Geometry: see drawing. Coordinates: mm, zero at the bounding-box minimum. Give positions to 0.01 mm unless a question says otherwise; leave off trailing zeros. Order: outer loops, then holes, each group sorted by start corner. A loop starts at its lowest first (then second) coordinate and runs counter-clockwise, first axis right, second up. Notation, with made-up numbers: (36, 62.25) -> (49, 62.25) arc R32 cw to (49, 91.25) -> close; hole circle Ø6 at (3, -3.5). An arc over 180 degrees is marked (long way). One line per item, written item: value. Start each with the question number.
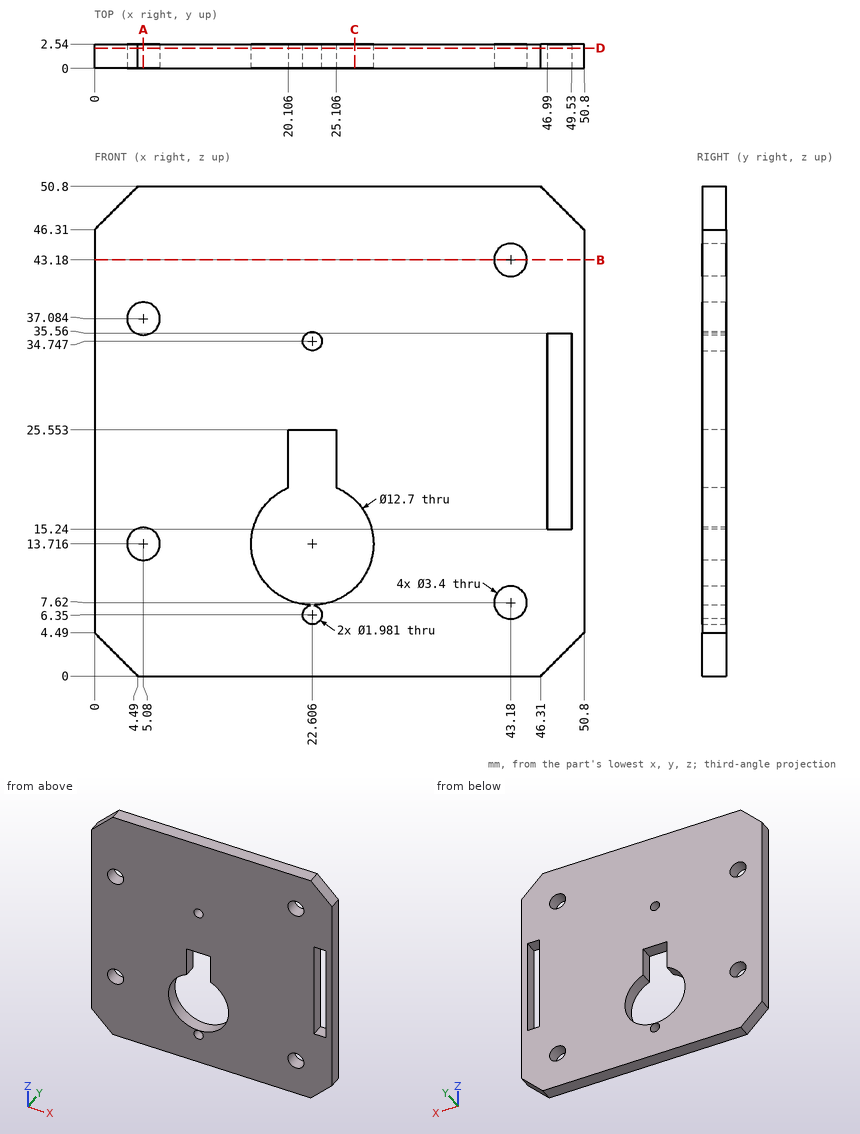
1. Cut plane A-A, the plane x = 5.08. Return loops of the section in (y, z).
2. Pin query (flat end, axial travel): P1, Ø0.8, axis at x = 48.5, y = 1, coming from the +Z side. Return the tip coordinate at first contact, or that it passes through.
3. Cut plane B-B, the plane z = 43.18. Return loops of the section in (x, y).
4. Cut plane C-C, the plane x = 27. Return loops of the section in (y, z).
5. Cut plane D-D, the plane y = 2.1. State how many separate pieces and enclosed holes the cut face has, then the cut area to 3 significant figures.
6. Material intervals for L1, parallel to X at y = 0.7, z = 13.5; L2, parallel to Z at x = 5.08, y = 1.55; L3, parallel to X at y = 0.35, z = 6.5 (1 decimal), sorted ascending. Write a range as [from, to].
Answers follow:
1. outline: (0, 0) -> (2.54, 0) -> (2.54, 12.02) -> (0, 12.02) -> close; (0, 15.42) -> (2.54, 15.42) -> (2.54, 35.38) -> (0, 35.38) -> close; (0, 38.78) -> (2.54, 38.78) -> (2.54, 50.8) -> (0, 50.8) -> close
2. P1: stops at z = 49.01
3. outline: (0, 0) -> (41.48, 0) -> (41.48, 2.54) -> (0, 2.54) -> close; (44.88, 0) -> (50.8, 0) -> (50.8, 2.54) -> (44.88, 2.54) -> close
4. outline: (0, 0) -> (2.54, 0) -> (2.54, 9.13) -> (0, 9.13) -> close; (0, 18.3) -> (2.54, 18.3) -> (2.54, 50.8) -> (0, 50.8) -> close
5. separate pieces: 1
5. enclosed holes: 8
5. area: 2,290 mm²
6. L1: x = [0, 3.39], [6.77, 16.26], [28.95, 50.8]
6. L2: z = [0, 12.02], [15.42, 35.38], [38.78, 50.8]
6. L3: x = [0, 21.6], [23.6, 41.9], [44.5, 50.8]
